```python
from build123d import *

# Parameters (mm, degrees)
SKETCH2_R           = 21.754264805
SKETCH2_W           = 8.5
SKETCH2_H           = 8.5
BOSS_EXTRUDE2_DEPTH = 15
FILLET2_R           = 5


with BuildPart() as part:
    # Sketch2 → Boss-Extrude2 (new body)
    with BuildSketch(Plane(origin=(0, 0, 0), x_dir=(1, 0, 0), z_dir=(0, 1, 0))):
        Polygon((184.942144259, 95.410610484), (89.679349842, 150.410610484), (89.679349842, 40.410610484), align=None)
        with Locations(Location((121.433614648, 95.410610484, 0), (0, 0, 270))):
            Circle(SKETCH2_R, mode=Mode.SUBTRACT)
        Polygon((105.484957808, 59.286726526), (98.123741876, 63.536726526), (93.873741876, 56.175510594), (101.234957808, 51.925510594), align=None, mode=Mode.SUBTRACT)
        with Locations((164.942144259, 95.410610484)):
            Rectangle(SKETCH2_W, SKETCH2_H, mode=Mode.SUBTRACT)
        Polygon((105.484957808, 131.534494442), (101.234957808, 138.895710374), (93.873741876, 134.645710374), (98.123741876, 127.284494442), align=None, mode=Mode.SUBTRACT)
    extrude(amount=BOSS_EXTRUDE2_DEPTH)

    # Fillet2
    fillet2_edges = [part.edges().sort_by_distance(p)[0] for p in [
        (89.679349842, 7.5, -40.410610484),
        (89.679349842, 7.5, -150.410610484),
        (184.942144259, 7.5, -95.410610484),
    ]]
    fillet(fillet2_edges, radius=FILLET2_R)


solid = part.part
```
CAD build for the part. Positions are in the model's coordinates, mm. A direction names the side the tool comes from. Coordinates: 2 decimals unless noted, no trailing zeros. Write each loop counter-clockwise with the first axis right and the second up, starting at its lowest first coordinate (ties: lowest second). Pieces come first, ordered by that corner, then holes. Notation, with made-up numbers: (51.5, 15.25) -> (72.5, 15.25) arc R26 cw to (72.5, 42.25) -> close; hole circle Ø1 at (15.25, 40.5). An arc over 180 degrees is marked (long way). Return JSON: item names as keys, results as strings. Group by question number.
Q1. Cut at D-D, the plane z = -92.5. Give the cut face in (x, y).
Q2. Which spindle directions (+Z, -Z, +X, -X, +Y, -Y) get a long thin tool onto all of the face, cutting with end or side? Do faces 5 (the face through (103.33, 7.395, -55.555)), 6 (the face through (92.243, 7.605, -44.705)). Say none if no direction does.
Q3. Flat gauge pins, fed straight in: pin 1 (2 mm diameter, centred on x = 167, y = 6, fed in from +Z); pin 2 (2.5 mm diameter, centred on x = 166, y = 5, fed in from -Z); pin 3 (4 mm diameter, centred on x = 112.5, y = 9, fed in from -Z). Where does each tip first touch, or does it go through?
Q4. Cut at B-B, the plane x = 117.5. Give the cut face in (y, z), then the cut area to 3 significant figures.
Q5. Cut at C-C, the plane y = 5.5. Give the cut face in (x, z), then the cut area to 3 significant figures.
Q6. Pull direction Z, two halves, no side cores. Call faces 1 (the face through (179.94, 7.6, -95.48)), 2 (the face through (102.134, 7.395, -85.372)), 3 (the face through (137.87, 7.4, -122.59)), 4 (the face through (101.75, 7.4, -129.38)): released by +Z, released by -Z, zero draft, split by the parting line, or undercut.
Q7. Cut at A-A, the plane z = -103.5. Give the cut face in (x, y).
Q8. Drill centre lines: line 1 (Z direction, x = 103, y = 14); line 2 (X direction, y = 12.75, z = -93); line 3 (Z direction, x = 96, y = 9.5). Where is each one in solid material? Low to high.
Returned:
{
 "1": {"outline": "(89.68, 0) -> (99.87, 0) -> (99.87, 15) -> (89.68, 15) -> close; (142.99, 0) -> (160.69, 0) -> (160.69, 15) -> (142.99, 15) -> close; (169.19, 0) -> (179.01, 0) -> (179.01, 15) -> (169.19, 15) -> close"},
 "2": {"face 5": "+Y, -Y", "face 6": "+Z, +Y, -Y"},
 "3": {"pin 1": "stops at z = -84.47", "pin 2": "stops at z = -107.07", "pin 3": "stops at z = -138.39"},
 "4": {"outline": "(0, -134.35) -> (15, -134.35) -> (15, -116.81) -> (0, -116.81) -> close; (0, -74.01) -> (15, -74.01) -> (15, -56.47) -> (0, -56.47) -> close", "area": "526 mm2"},
 "5": {"outline": "(89.68, -141.75) arc R5 ccw to (97.18, -146.08) -> (177.44, -99.74) arc R5 ccw to (177.44, -91.08) -> (97.18, -44.74) arc R5 ccw to (89.68, -49.07) -> close; hole (93.87, -134.65) -> (101.23, -138.9) -> (105.48, -131.53) -> (98.12, -127.28) -> close; hole (93.87, -56.18) -> (98.12, -63.54) -> (105.48, -59.29) -> (101.23, -51.93) -> close; hole circle Ø43.51 at (121.43, -95.41); hole (160.69, -99.66) -> (169.19, -99.66) -> (169.19, -91.16) -> (160.69, -91.16) -> close", "area": "3,480 mm2"},
 "6": {"face 1": "split by the parting line", "face 2": "undercut", "face 3": "released by -Z", "face 4": "undercut"},
 "7": {"outline": "(89.68, 0) -> (101.24, 0) -> (101.24, 15) -> (89.68, 15) -> close; (141.63, 0) -> (170.93, 0) -> (170.93, 15) -> (141.63, 15) -> close"},
 "8": {"line 1": "z = -142.72 to -135.84, -130.1 to -106.96, -83.86 to -60.72, -54.98 to -48.1", "line 2": "x = 89.68 to 99.81, 143.05 to 160.69, 169.19 to 179.32", "line 3": "z = -146.57 to -135.87, -130.96 to -59.86, -54.95 to -44.25"}
}
